Solid Edge part; units mm, degrees
sketch "Sketch1" plane through (0, 0, 0) normal (0, 0, 1) x (1, 0, 0)
  line L0 (-46, -29) -> (46, -29)
  line L1 (46, -29) -> (46, 29)
  line L2 (46, 29) -> (-46, 29)
  line L3 (-46, 29) -> (-46, -29)
  dimension "D1" = 46
  dimension "D2" = 46
extrude "Ajout_matière_1" add sketch "Sketch1" along normal mid plane 5
sketch "Sketch2" plane through (46, 0, 0) normal (1, 0, 0) x (0, 1, 0)
  circle A0 centre (0, -5.5) radius 6
extrude "Cutout1" cut sketch "Sketch2" against normal through all
hole "Perçage_1" at (-43.5, 26.5, 2.5) direction (0, 0, -1) diameter 3.1 end up to next
hole "Hole1" at (43.5, 26.5, 2.5) direction (0, 0, -1) diameter 3.1 end up to next
hole "Hole2" at (43.5, -26.5, 2.5) direction (0, 0, -1) diameter 3.1 end up to next
hole "Hole3" at (-43.5, -26.5, 2.5) direction (0, 0, -1) diameter 3.1 end up to next
hole "Hole4" at (-36, -22.87, 2.5) direction (0, 0, -1) diameter 1.8 end up to next
hole "Hole5" at (-36, 24.13, 2.5) direction (0, 0, -1) diameter 1.8 end up to next
hole "Hole6" at (-24.6, 24.13, 2.5) direction (0, 0, -1) diameter 1.8 end up to next
hole "Hole7" at (-24.6, -22.87, 2.5) direction (0, 0, -1) diameter 1.8 end up to next
hole "Perçage_13" at (-14.6642, -9, 2.5) direction (0, 0, -1) diameter 2.8 end up to next
hole "Hole8" at (34.6858, 17.4, 2.5) direction (0, 0, -1) diameter 2.8 end up to next
hole "Hole9" at (-7.3142, 17.4, 2.5) direction (0, 0, -1) diameter 2.8 end up to next
hole "Hole10" at (42, -9, 2.5) direction (0, 0, -1) diameter 2.8 end up to next
properties material "Plastique ABS, performance moyenne"
Part model, mm, in its own coordinate system. Give positions to 0.01 mm unless a question says otherwise; leave off trailing zeros. Write each loop counter-clockwise with the first axis right and the second up, starting at its lowest first coordinate (ties: lowest second). Pieces come first, ordered by that corner, then holes. Notation, with made-up numbers: M -38,31.5 L -10,31.5 A17 cw -10,38.5 Z; hole C 23,38 d3. An arc over 180 degrees is marked long. Use CSV: the item, a comma, the result in double quotes.
Item 1: Slice it at A-A on x = -24.6. Write the cut outline in (y, z), plus the area to 3 significant figures.
Taken from the geometry:
outline,"M -29,-2.5 L -23.77,-2.5 L -23.77,2.5 L -29,2.5 Z; M -21.97,-2.5 L -5.2,-2.5 A6 cw 5.2,-2.5 L 23.23,-2.5 L 23.23,2.5 L -21.97,2.5 Z; M 25.03,-2.5 L 29,-2.5 L 29,2.5 L 25.03,2.5 Z"
area,"250 mm²"
Item 2: Drill centre lines: probe 1 along Y at (x, z) = (43.5, 1.4); probe 2 along Y at (x, z) = (-36, 2.2); probe 3 along X at (y, z) = (-26, -1.5). Where is each one in solid material? Low to high.
Taken from the geometry:
probe 1,"y = -29 to -28.05, -24.95 to 24.95, 28.05 to 29"
probe 2,"y = -29 to -23.77, -21.97 to 23.23, 25.03 to 29"
probe 3,"x = -46 to -44.97, -42.03 to 42.03, 44.97 to 46"
Item 3: Slice it at D-D on y = 17.4. Write the cut outline in (x, z), plus the area to 3 significant figures.
Taken from the geometry:
outline,"M -46,-2.5 L -8.71,-2.5 L -8.71,2.5 L -46,2.5 Z; M -5.91,-2.5 L 33.29,-2.5 L 33.29,2.5 L -5.91,2.5 Z; M 36.09,-2.5 L 46,-2.5 L 46,2.5 L 36.09,2.5 Z"
area,"432 mm²"
Item 4: Slice it at B-B on y = -26.5. Write the cut outline in (x, z), plus the area to 3 significant figures.
Taken from the geometry:
outline,"M -46,-2.5 L -45.05,-2.5 L -45.05,2.5 L -46,2.5 Z; M -41.95,-2.5 L 41.95,-2.5 L 41.95,2.5 L -41.95,2.5 Z; M 45.05,-2.5 L 46,-2.5 L 46,2.5 L 45.05,2.5 Z"
area,"429 mm²"
Item 5: Slice it at C-C on z = -0.35. State how many separate pieces and enclosed holes the cut face has, plus the area to 3 significant figures.
Taken from the geometry:
separate pieces,"2"
enclosed holes,"12"
area,"4,700 mm²"
Item 6: Pull direction X, two halves, no side cores. Call faces 1 (the face through (-1, 17, -2.5)), 2 (the face through (-23.71, 24.25, 0.04)), 3 (the face through (-46, 0, 1)): +X half, -X half, draft (parallel to the pull), parting line (faces both ways), or undercut.
Taken from the geometry:
face 1,"draft"
face 2,"undercut"
face 3,"-X half"
